Geometry check sheet. Reference: the model listing, model coordinates, mm. Face numbers are marked on the shaded views. A direction names the side the tool comes from. Round coordinates to 2 decimals unless told otherwise and drop trailing zeros. Loops run counter-clockwise (first coordinate to the right, second up) from the corner with the lowest first, then second, coordinate; pieces in that order, holes last. Notation, with made-up numbers: M -3.5,37 L 8.5,37 A20 ccw 8.5,55 Z; hole C -7,39.25 d8. An arc over 180 degrees is marked long. Write item = value, one per line.
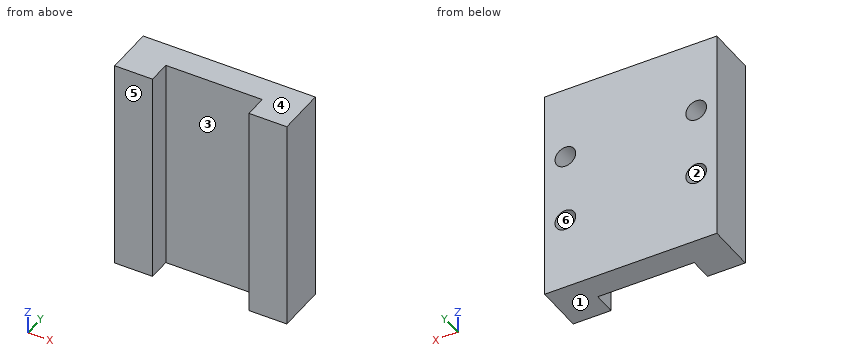
from build123d import *

# Parameters (mm, degrees)
SKETCH_1_W               = 25
SKETCH_1_H               = 7.1
EXTRUDE_1_DEPTH          = 15.6
CUT_EXTRUDE_1_DEPTH      = 34.797817977
CUT_EXTRUDE_1_DEPTH_BACK = 34.797817977
SKETCH_2_W               = 14
SKETCH_2_H               = 3.3
SKETCH_3_R               = 1.5
CUT_EXTRUDE_2_DEPTH      = 3


with BuildPart() as part:
    # 草图1 → 凸台-拉伸1 (new, symmetric)
    with BuildSketch(Plane.XY):
        Rectangle(SKETCH_1_W, SKETCH_1_H)
    extrude(amount=EXTRUDE_1_DEPTH, both=True)

    # 草图2 → 切除-拉伸1 (cut, two sides: drawn at the far end of the back side and taken through both)
    with BuildSketch(Plane.XY.offset(15.6).offset(-CUT_EXTRUDE_1_DEPTH_BACK)):
        with Locations((0, -1.9)):
            Rectangle(SKETCH_2_W, SKETCH_2_H)
    extrude(amount=CUT_EXTRUDE_1_DEPTH + CUT_EXTRUDE_1_DEPTH_BACK, mode=Mode.SUBTRACT)

    # 草图3 → 切除-拉伸2 (cut)
    with BuildSketch(Plane(origin=(0, 3.55, 0), x_dir=(1, 0, 0), z_dir=(0, 1, 0))):
        with Locations(Location((9.5, -5, 0), (0, 0, 270))):
            Circle(SKETCH_3_R)
        with Locations(Location((-9.5, -5, 0), (0, 0, 270))):
            Circle(SKETCH_3_R)
        with Locations(Location((-9.5, 5, 0), (0, 0, 270))):
            Circle(SKETCH_3_R)
        with Locations(Location((9.5, 5, 0), (0, 0, 270))):
            Circle(SKETCH_3_R)
    extrude(amount=-CUT_EXTRUDE_2_DEPTH, mode=Mode.SUBTRACT)


solid = part.part
(1) Tool access check on the marked faces 1, 2 and 3. Record the directions out of +Z, -Z, +X, -X, +Y, -Y that give a thin tool (end or side, any length) a straight path to the whole face; none if there is none.
Result set:
face_1 = -Z, +X, -X, +Y, -Y
face_2 = +Y
face_3 = +Z, -Z, -Y
(2) Sectioned sample at B-B on y = 1.75. Record the cut outline in (x, z), then the cut area to 3 significant figures.
Result set:
outline = M -12.5,-15.6 L 12.5,-15.6 L 12.5,15.6 L -12.5,15.6 Z; hole C -9.5,-5 d3; hole C -9.5,5 d3; hole C 9.5,-5 d3; hole C 9.5,5 d3
area = 752 mm2
(3) Sectioned sample at A-A on y = -1.75. Record the cut outline in (x, z).
Result set:
outline = M -12.5,-15.6 L -7,-15.6 L -7,15.6 L -12.5,15.6 Z; M 7,-15.6 L 12.5,-15.6 L 12.5,15.6 L 7,15.6 Z
(4) Sectioned sample at C-C on x = -9.5. Record the cut outline in (y, z), then the cut area to 3 significant figures.
Result set:
outline = M -3.55,-15.6 L 3.55,-15.6 L 3.55,-6.5 L 0.55,-6.5 L 0.55,-3.5 L 3.55,-3.5 L 3.55,3.5 L 0.55,3.5 L 0.55,6.5 L 3.55,6.5 L 3.55,15.6 L -3.55,15.6 Z
area = 204 mm2
(5) Release check for a two-part mould opening along Z. For the marked faces 4, 5 and 6 record: released by +Z, released by -Z, zero draft, split by the parting line, or undercut.
Result set:
face_4 = released by +Z
face_5 = zero draft
face_6 = undercut
(6) Depth check by flat-ended pin: pin 1 Ø0.9 at (x, z) = (-9, -5.5) entering from +Y; pin 2 Ø4 at (x, z) = (-2.5, -4.5) entering from -Y. Enter the tip coordinate at first touch or a pass-through.
Result set:
pin_1 = 0.55
pin_2 = -0.25
(7) Material ranges on line 1 along X through (y, z) = (2.15, 5); line 2 along X through (y, z) = (-2, 10.5); line 3 along Y through (x, z) = (-1, 3.5), recorded low to high. Write a range as from..to.
Result set:
line_1 = -12.5..-11, -8..8, 11..12.5
line_2 = -12.5..-7, 7..12.5
line_3 = -0.25..3.55
(8) Sectioned sample at D-D on z = -5. Record the cut outline in (x, y).
Result set:
outline = M -12.5,-3.55 L -7,-3.55 L -7,-0.25 L 7,-0.25 L 7,-3.55 L 12.5,-3.55 L 12.5,3.55 L 11,3.55 L 11,0.55 L 8,0.55 L 8,3.55 L -8,3.55 L -8,0.55 L -11,0.55 L -11,3.55 L -12.5,3.55 Z
